Verification items for the finished model (mm, model axes). Face numbers are marked on the shaded views. A direction names the side the tool comes from. Round coordinates to 2 decimals unless told otherwise and drop trailing zeros. Order: outer loops, then holes, each group sorted by start corner. A loop starts at its lowest first (then second) coordinate and runs counter-clockwise, first axis right, second up. Notation, with made-up numbers: M 21.25,39.25 L 38.25,39.25 A14 cw 38.25,48.25 Z; hole C -22.75,-13.5 d6. An arc over 180 degrees is marked long. Use one line per item in the form item = value. Start each with the question number.
Item 1: Cross-section at C-C on x = -30. Enter the section's corners in (y, z), then the cut area to 3 significant figures.
Item 2: Cross-section at A-A on z = 17.75. Enter the section's corners in (x, y).
Item 3: Release check for a two-part mould opening along Y. For the marked faces 1, 2, 3 and 4 record: +Y half, -Y half, draft (parallel to the pull), parting line (faces both ways), or undercut.
Item 4: Cross-section at D-D on y = -26.5. Enter the section's corners in (x, z).
Item 5: Thickness scan on probe 1 along Y at (x, z) = (0, 14.5); probe 2 along X at (y, z) = (0, 10); probe 3 along Y at (x, z) = (15, 4.5). Record the ranges inside material, lowest first. Write a range as [from, to].
Item 6: Cross-section at B-B on y = 0. Enter the section's corners in (x, z), then the cut area to 3 significant figures.
Item 7: Go/stop test with flat-tipped pins: pin 1 Ø10 at (x, z) = (55.5, 12.5) entering from +Y; pin 2 Ø10 at (y, z) = (-4.5, 12.5) entering from -X; pin 3 Ø3 at (x, z) = (38.5, 3.5) entering from +Y. Record where each tip stops, or that it passes through.
Item 8: Tool access check on the marked faces 5 and 6. Record the directions out of +Z, -Z, +X, -X, +Y, -Y that give a thin tool (end or side, any length) a straight path to the whole face; none if there is none.
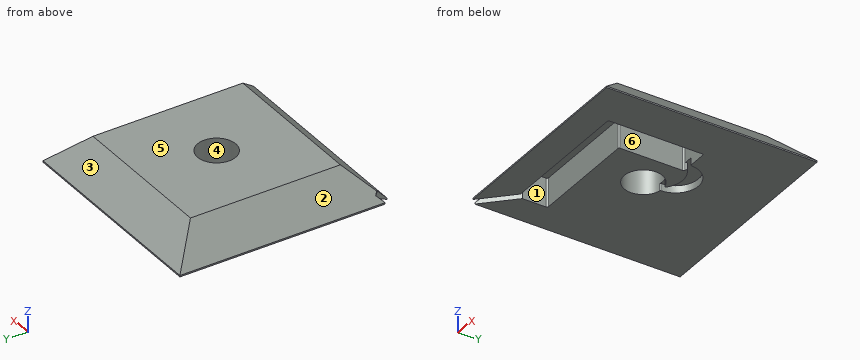
from build123d import *

# Parameters (mm, degrees)
SKETCH_W        = 146
SKETCH_H        = 146
PAD_DEPTH       = 22
CHAMFER_SIZE    = 21
SKETCH001_R     = 13.25
POCKET_DEPTH    = 22.001
SKETCH002_W     = 21
SKETCH002_H     = 66.25
SKETCH002_W_2   = 76
SKETCH002_H_2   = 21
POCKET001_DEPTH = 20
POCKET002_DEPTH = 5
POCKET003_DEPTH = 22.001
FILLET_R        = 1
FILLET001_R     = 0.7


with BuildPart() as part:
    # Sketch → Pad (new body)
    with BuildSketch(Plane.XY):
        Rectangle(SKETCH_W, SKETCH_H)
    extrude(amount=PAD_DEPTH)

    # Chamfer
    chamfer_edges = [part.edges().sort_by_distance(p)[0] for p in [
        (73, 0, 22),
        (0, -73, 22),
        (-73, 0, 22),
        (0, 73, 22),
    ]]
    chamfer(chamfer_edges, length=CHAMFER_SIZE)

    # Sketch001 (on Face6 of Pad) → Pocket (cut, through all)
    with BuildSketch(Plane.XY.offset(22)):
        Circle(SKETCH001_R)
    extrude(amount=-POCKET_DEPTH, mode=Mode.SUBTRACT)

    # Sketch002 (on Face4 of Pocket) → Pocket001 (cut)
    with BuildSketch(Plane(origin=(0, 0, 0), x_dir=(1, 0, 0), z_dir=(0, 0, -1))):
        with Locations((33.5, 19.875)):
            Rectangle(SKETCH002_W, SKETCH002_H)
        with Locations((-15, 42.5)):
            Rectangle(SKETCH002_W_2, SKETCH002_H_2)
    extrude(amount=-POCKET001_DEPTH, mode=Mode.SUBTRACT)

    # Sketch003 (on Face4 of Pocket001) → Pocket002 (cut)
    with BuildSketch(Plane(origin=(0, 0, 0), x_dir=(1, 0, 0), z_dir=(0, 0, -1))):
        with BuildLine():
            Line((26, -13.25), (30, -13.25))
            ThreePointArc((-2, -13.098187), (13.924093, -29.174093), (30, -13.25))
            Line((2, -13.098187), (-2, -13.098187))
            ThreePointArc((2, -13.098187), (13.968558, -18.144656), (26, -13.25))
        make_face()
        Polygon((-49.464466, 53), (-71.232233, 74.767767), (-74.767767, 71.232233), (-53, 49.464466), align=None)
    extrude(amount=-POCKET002_DEPTH, mode=Mode.SUBTRACT)

    # Sketch004 (on Face3 of Pocket002) → Pocket003 (cut, through all)
    with BuildSketch(Plane(origin=(0, 0, 0), x_dir=(1, 0, 0), z_dir=(0, 0, -1))):
        Polygon((-69, 65.464466), (-65.464466, 69), (-69.464466, 73), (-73, 69.464466), align=None)
    extrude(amount=-POCKET003_DEPTH, mode=Mode.SUBTRACT)

    # Fillet
    fillet_edges = [part.edges().sort_by_distance(p)[0] for p in [
        (-53, -32, 10),
        (23, -32, 10),
        (23, 13.25, 10),
        (44, -53, 10),
        (44, 13.25, 10),
        (-53, -53, 12.5),
    ]]
    fillet(fillet_edges, radius=FILLET_R)

    # Fillet001
    fillet001_edges = [part.edges().sort_by_distance(p)[0] for p in [
        (2, 13.098187, 2.5),
        (30, 13.25, 2.5),
        (26, 13.25, 2.5),
        (-2, 13.098187, 2.5),
    ]]
    fillet(fillet001_edges, radius=FILLET001_R)


solid = part.part
Output values:
q1.outline = M -73,0 L -53,0 L -53,20 L -32,20 L -32,0 L 73,0 L 73,1 L 52,22 L -52,22 L -73,1 Z
q1.area = 2,350 mm2
q2.outline = M -56.25,-56.25 L 56.25,-56.25 L 56.25,56.25 L -56.25,56.25 Z; hole M -53,-52 A1 ccw -52,-53 L 43,-53 A1 ccw 44,-52 L 44,12.25 A1 ccw 43,13.25 L 24,13.25 A1 ccw 23,12.25 L 23,-31 A1 cw 22,-32 L -52,-32 A1 ccw -53,-33 Z; hole C 0,0 d26.5
q3.face_1 = undercut
q3.face_2 = draft
q3.face_3 = +Y half
q3.face_4 = undercut
q4.outline = M -73,0 L 23,0 L 23,20 L 44,20 L 44,0 L 73,0 L 73,1 L 52,22 L -52,22 L -73,1 Z
q5.probe_1 = [-59.5, -53], [-32, -13.25], [13.25, 59.5]
q5.probe_2 = [-64, -13.25], [13.25, 23], [44, 64]
q5.probe_3 = [-69.5, -53], [-32, 18.12], [29.14, 69.5]
q6.outline = M -73,0 L -13.25,0 L -13.25,22 L -52,22 L -73,1 Z; M 13.25,0 L 23,0 L 23,20 L 44,20 L 44,0 L 73,0 L 73,1 L 52,22 L 13.25,22 Z
q6.area = 1,770 mm2
q7.pin_1 = 66.5
q7.pin_2 = -66.5
q7.pin_3 = 72
q8.face_5 = +Z, +X, -X, +Y, -Y
q8.face_6 = -Z
